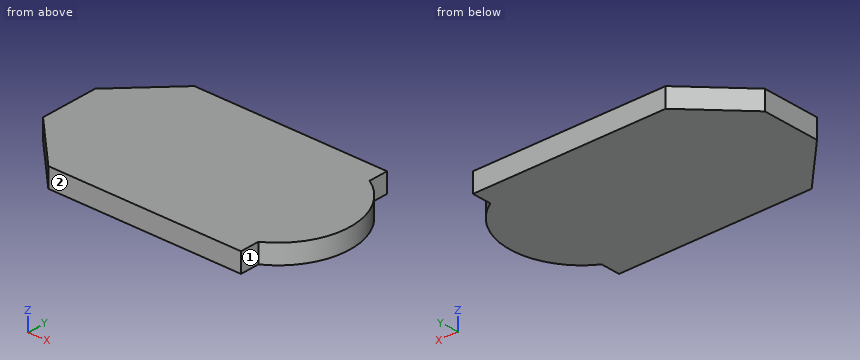
from build123d import *

# Parameters (mm, degrees)
SM_BASE_FLANGE_1_DEPTH = 5


# Sheet-metal steps are written as plain solids
with BuildPart() as part:
    # Sketch 1 → Базовая кромка1 (new body)
    with BuildSketch(Plane.XY):
        with BuildLine():
            Line((29.76239566, 16.000000043), (29.76239566, 21.000000043))
            Line((29.76239566, 21.000000043), (-20, 21.000000043))
            Line((-20, 21.000000043), (-33.500000043, 7.5))
            Line((-33.500000043, 7.5), (-33.500000043, -7.5))
            Line((-33.500000043, -7.5), (-20, -21.000000043))
            Line((-20, -21.000000043), (29.76239566, -21.000000043))
            Line((29.76239566, -21.000000043), (29.76239566, -16.000000043))
            ThreePointArc((29.76239566, -16.000000043), (39.00000001, -1.1e-08), (29.76239566, 16.000000043))
        make_face()
    extrude(amount=-SM_BASE_FLANGE_1_DEPTH)


solid = part.part
Input: part model. Units: mm. Frame: model coordinates. Face numbers are marked on the shaded views. A direction names the side the tool comes from. Coordinates: 2 decimals unless noted, no trailing zeros. Loops run counter-clockwise (first coordinate to the right, second up) from the corner with the lowest first, then second, coordinate; pieces in that order, holes last.
(1) Section B-B on x = -24. Return the cut outline in (y, z), then the cut area to 3 significant figures.
(2) Material intervals for probe 1 along X at (y, z) = (-2, -3.2); probe 2 along Y at (x, z) = (-25.5, -2.4); probe 3 along X at (y, z) = (-0.5, -4.15), sorted ascending.
(3) First-contact query: pin 1 Ø1.5 at (y, z) = (18, -1.5) entering from +X; pin 2 Ø1 at (y, z) = (11, -4.5) entering from +X. Flat tips, straight axial feed; report the tip coordinate or a pass-through.
(4) Set-up query: the marked faces 1 and 2. Return all of +Z, -Z, +X, -X, +Y, -Y with unobstructed straight access to the full face (end or side cutting, diameter ignored); none if empty.
(5) Section A-A on z = -4.15. Return the cut outline in (x, y).
(6) Section C-C on y = -9.5. Return the cut outline in (x, z).
Data:
1. outline: (-17, -5) - (17, -5) - (17, 0) - (-17, 0) - close
1. area: 170 mm2
2. probe 1: x = -33.5 to 38.89
2. probe 2: y = -15.5 to 15.5
2. probe 3: x = -33.5 to 38.99
3. pin 1: stops at x = 29.76
3. pin 2: stops at x = 35.73
4. face 1: +Z, -Z, +X, -Y
4. face 2: +Z, -Z, +X, -X, -Y
5. outline: (-33.5, -7.5) - (-20, -21) - (29.76, -21) - (29.76, -16) arc R18.48 ccw to (29.76, 16) - (29.76, 21) - (-20, 21) - (-33.5, 7.5) - close
6. outline: (-31.5, -5) - (36.37, -5) - (36.37, 0) - (-31.5, 0) - close
